```python
from build123d import *

# Parameters (mm, degrees)
SKETCH1_W           = 104.672897196
SKETCH1_H           = 66.728971962
SKETCH1_R           = 2
SKETCH1_R_2         = 1.5
BOSS_EXTRUDE1_DEPTH = 3


with BuildPart() as part:
    # Sketch1 → Boss-Extrude1 (new body)
    with BuildSketch(Plane(origin=(0, 0, 0), x_dir=(1, 0, 0), z_dir=(0, 1, 0))):
        Rectangle(SKETCH1_W, SKETCH1_H)
        with Locations(Location((35, 0, 0), (0, 0, 270))):
            Circle(SKETCH1_R, mode=Mode.SUBTRACT)
        with Locations(Location((15, 0, 0), (0, 0, 270))):
            Circle(SKETCH1_R, mode=Mode.SUBTRACT)
        with Locations(Location((-15, 0, 0), (0, 0, 270))):
            Circle(SKETCH1_R, mode=Mode.SUBTRACT)
        with Locations(Location((-47.336448598, 28.364485981, 0), (0, 0, 270))):
            Circle(SKETCH1_R_2, mode=Mode.SUBTRACT)
        with Locations(Location((47.336448598, 28.364485981, 0), (0, 0, 90))):
            Circle(SKETCH1_R_2, mode=Mode.SUBTRACT)
        with Locations(Location((-47.336448598, -28.364485981, 0), (0, 0, 90))):
            Circle(SKETCH1_R_2, mode=Mode.SUBTRACT)
        with Locations(Location((47.336448598, -28.364485981, 0), (0, 0, 270))):
            Circle(SKETCH1_R_2, mode=Mode.SUBTRACT)
        with BuildLine():
            Line((40.629165125, -3.25), (45.836448598, -3.25))
            Line((45.836448598, -3.25), (45.836448598, -22.039930661))
            ThreePointArc((45.836448598, -22.039930661), (42.74025452, -23.768291904), (41.011893278, -26.864485981))
            Line((41.011893278, -26.864485981), (18.25, -26.864485981))
            Line((18.25, -26.864485981), (18.25, -5.629165125))
            ThreePointArc((18.25, -5.629165125), (19.596194078, -4.596194078), (20.629165125, -3.25))
            Line((20.629165125, -3.25), (29.370834875, -3.25))
            ThreePointArc((29.370834875, -3.25), (35, -6.5), (40.629165125, -3.25))
        make_face(mode=Mode.SUBTRACT)
        with BuildLine():
            Line((-18.25, -26.864485981), (-18.25, -5.629165125))
            ThreePointArc((-18.25, -5.629165125), (-19.596194078, -4.596194078), (-20.629165125, -3.25))
            Line((-20.629165125, -3.25), (-45.836448598, -3.25))
            Line((-45.836448598, -3.25), (-45.836448598, -22.039930661))
            ThreePointArc((-45.836448598, -22.039930661), (-42.74025452, -23.768291904), (-41.011893278, -26.864485981))
            Line((-41.011893278, -26.864485981), (-18.25, -26.864485981))
        make_face(mode=Mode.SUBTRACT)
        with BuildLine():
            Line((-11.75, -26.864485981), (-11.75, -5.629165125))
            ThreePointArc((-11.75, -5.629165125), (-10.403805922, -4.596194078), (-9.370834875, -3.25))
            Line((-9.370834875, -3.25), (9.370834875, -3.25))
            ThreePointArc((9.370834875, -3.25), (10.403805922, -4.596194078), (11.75, -5.629165125))
            Line((11.75, -5.629165125), (11.75, -26.864485981))
            Line((11.75, -26.864485981), (-11.75, -26.864485981))
        make_face(mode=Mode.SUBTRACT)
        with BuildLine():
            Line((40.629165125, 3.25), (45.836448598, 3.25))
            Line((45.836448598, 3.25), (45.836448598, 22.039930661))
            ThreePointArc((45.836448598, 22.039930661), (42.74025452, 23.768291904), (41.011893278, 26.864485981))
            Line((41.011893278, 26.864485981), (18.25, 26.864485981))
            Line((18.25, 26.864485981), (18.25, 5.629165125))
            ThreePointArc((18.25, 5.629165125), (19.596194078, 4.596194078), (20.629165125, 3.25))
            Line((20.629165125, 3.25), (29.370834875, 3.25))
            ThreePointArc((29.370834875, 3.25), (35, 6.5), (40.629165125, 3.25))
        make_face(mode=Mode.SUBTRACT)
        with BuildLine():
            Line((-11.75, 26.864485981), (11.75, 26.864485981))
            Line((11.75, 26.864485981), (11.75, 5.629165125))
            ThreePointArc((11.75, 5.629165125), (10.403805922, 4.596194078), (9.370834875, 3.25))
            Line((9.370834875, 3.25), (-9.370834875, 3.25))
            ThreePointArc((-9.370834875, 3.25), (-10.403805922, 4.596194078), (-11.75, 5.629165125))
            Line((-11.75, 5.629165125), (-11.75, 26.864485981))
        make_face(mode=Mode.SUBTRACT)
        with BuildLine():
            Line((-45.836448598, 3.25), (-20.629165125, 3.25))
            ThreePointArc((-20.629165125, 3.25), (-19.596194078, 4.596194078), (-18.25, 5.629165125))
            Line((-18.25, 5.629165125), (-18.25, 26.864485981))
            Line((-18.25, 26.864485981), (-41.011893278, 26.864485981))
            ThreePointArc((-41.011893278, 26.864485981), (-42.74025452, 23.768291904), (-45.836448598, 22.039930661))
            Line((-45.836448598, 22.039930661), (-45.836448598, 6.771875217))
            Line((-45.836448598, 6.771875217), (-45.836448598, 3.25))
        make_face(mode=Mode.SUBTRACT)
    extrude(amount=BOSS_EXTRUDE1_DEPTH)


solid = part.part
```
The model under review builds one solid part; all positions refer to its coordinate system, in mm. Round coordinates to 2 decimals unless told otherwise and drop trailing zeros. Loops run counter-clockwise (first coordinate to the right, second up) from the corner with the lowest first, then second, coordinate; pieces in that order, holes last. Notation, with made-up numbers: (7.5, 58) - (27.5, 58) arc R26 cw to (27.5, 75) - close; hole circle Ø5 at (89.5, 21). An arc over 180 degrees is marked (long way). Use a Markdown table: item, result. Add a question column.
Q1. The part is to be moulded in two halves that separate along Z. For faces 1 (the face through (-12, 3, 0)), 2 (the face through (34.9, 1.5, -6.5)), say which applies: pulls with the +Z half, pulls with the -Z half, needs draft (parallel to the pull), parting line crosses it, or undercut.
Q2. Add section D-D (z = 28). State the section outline as (x, y) points.
Q3. Add section A-A (x = 0.5). State the section outline as (y, z) points, plus the area to 3 significant figures.
Q4. Add section C-C (x = -15). State the section outline as (y, z) points, plus the area to 3 significant figures.
Q5. For probe 1 along X at (y, z) = (2.25, 9); probe 2 along Z at (x, y) = (7, 1.6), list the stretches that pass through material, from the lowest coordinate up.
Q6. Add section B-B (z = -16.5). State the section outline as (x, y) points.
Worked answers:
| question | item | result |
|---|---|---|
| 1 | face 1 | needs draft |
| 1 | face 2 | undercut |
| 2 | outline | (-52.34, 0) - (-48.79, 0) - (-48.79, 3) - (-52.34, 3) - close; (-45.88, 0) - (45.88, 0) - (45.88, 3) - (-45.88, 3) - close; (48.79, 0) - (52.34, 0) - (52.34, 3) - (48.79, 3) - close |
| 3 | outline | (0, -33.36) - (3, -33.36) - (3, -26.86) - (0, -26.86) - close; (0, -3.25) - (3, -3.25) - (3, 3.25) - (0, 3.25) - close; (0, 26.86) - (3, 26.86) - (3, 33.36) - (0, 33.36) - close |
| 3 | area | 58.5 mm² |
| 4 | outline | (0, -33.36) - (3, -33.36) - (3, -2) - (0, -2) - close; (0, 2) - (3, 2) - (3, 33.36) - (0, 33.36) - close |
| 4 | area | 188 mm² |
| 5 | probe 1 | -52.34 to -45.84, -18.25 to -11.75, 11.75 to 18.25, 45.84 to 52.34 |
| 5 | probe 2 | -33.36 to -26.86, -3.25 to 3.25, 26.86 to 33.36 |
| 6 | outline | (-52.34, 0) - (-45.84, 0) - (-45.84, 3) - (-52.34, 3) - close; (-18.25, 0) - (-11.75, 0) - (-11.75, 3) - (-18.25, 3) - close; (11.75, 0) - (18.25, 0) - (18.25, 3) - (11.75, 3) - close; (45.84, 0) - (52.34, 0) - (52.34, 3) - (45.84, 3) - close |
